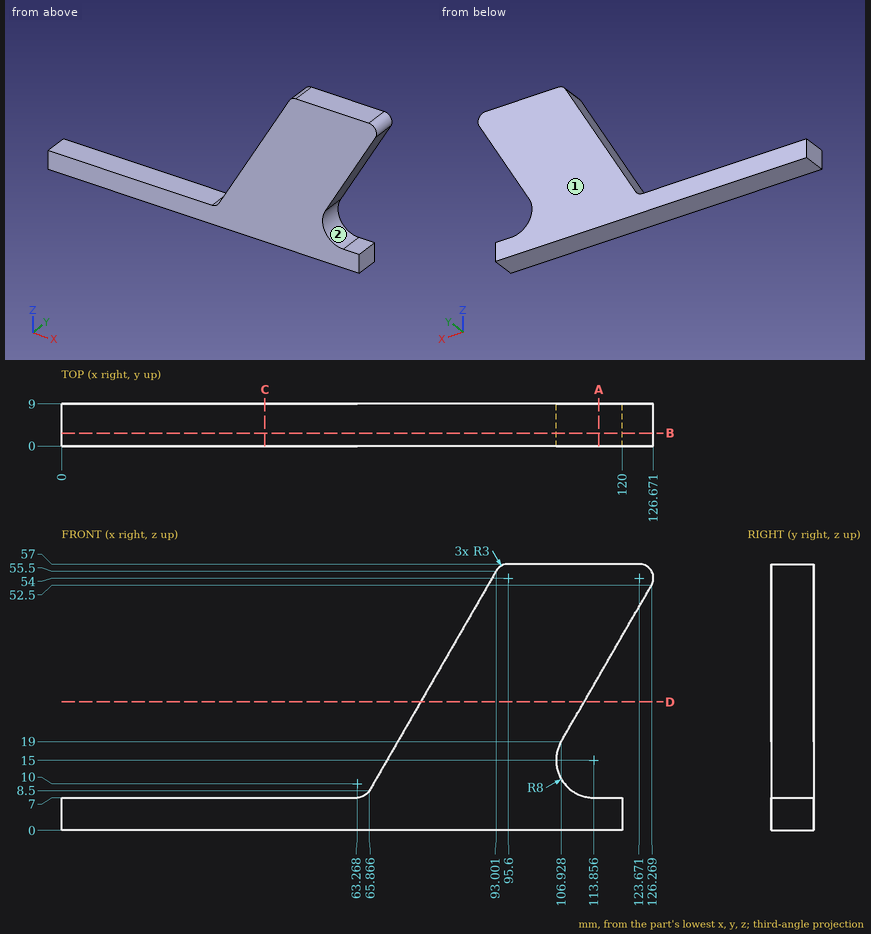
Print and shaded views of the part. All mm, measured from the part's lowest x, y and z. Coordinates: 2 decimals unless noted, no trailing zeros. Loops run counter-clockwise (first coordinate to the right, second up) from the corner with the lowest first, then second, coordinate; pieces in that order, holes last. Notation, with made-up numbers: M 60,-12 L 90,-12 A19 ccw 90,24 Z; hole C 8,-4 d10. An arc over 180 degrees is marked long. Use a Markdown table: item, result. Add a question column.
Q1. Cut at D-D (z = 27.5). Write the cut outline in (x, y) (1 decimal), and give its area (3 significant figures).
Q2. Cut at B-B (y = 2.75). Write the cut outline in (x, z).
Q3. Mould opens along Z. For the marked faces 1 and 2 say: +Z half, -Z half, draft (parallel to the pull), parting line (faces both ways), or undercut.
Q4. Cut at A-A (x = 115). Write the cut outline in (y, z), and give its area (3 significant figures).
Q5. Probe L1, parallel to Z at x = 36, y = 0.75; L2, parallel to X at y = 4, z = 5.5; L3, parallel to Z at x = 110, y = 6.75 (1 decimal). List the from-to ranges inside material, lowest first.
Q6. Cut at C-C (x = 43.5). Write the cut outline in (y, z).
Worked out:
| question | item | result |
|---|---|---|
| 1 | outline | M 76.8,0 L 111.8,0 L 111.8,9 L 76.8,9 Z |
| 1 | area | 315 mm2 |
| 2 | outline | M 0,0 L 120,0 L 120,7 L 113.86,7 A8 cw 106.93,19 L 126.27,52.5 A3 ccw 123.67,57 L 95.6,57 A3 ccw 93,55.5 L 65.87,8.5 A3 cw 63.27,7 L 0,7 Z |
| 3 | face 1 | draft |
| 3 | face 2 | undercut |
| 4 | outline | M 0,0 L 9,0 L 9,7 L 0,7 Z; M 0,32.98 L 9,32.98 L 9,57 L 0,57 Z |
| 4 | area | 279 mm2 |
| 5 | L1 | z = 0 to 7 |
| 5 | L2 | x = 0 to 120 |
| 5 | L3 | z = 0 to 8, 24.3 to 57 |
| 6 | outline | M 0,0 L 9,0 L 9,7 L 0,7 Z |
